Drawing for the job (mm, zero at the part's lowest x, y, z). A direction names the side the tool comes from. Round coordinates to 2 decimals unless told otherwise and drop trailing zeros. Write each loop counter-clockwise with the first axis right and the second up, starting at its lowest first coordinate (ties: lowest second). Pieces come first, ordered by that corner, then holes.
Item 1: Band-saw the part on C-C, the plane z = 1.25. Write the cut outline in (x, y).
Item 2: Drop flat-ended pins along their axis: pin 1 Ø3 at (y, z) = (3.5, 6) entering from +X; pin 2 Ø1.5 at (x, z) = (3.5, 4.5) entering from -Y; pin 3 Ø3 at (y, z) = (3, 9) entering from -X. Give the stop position or say it passes through.
Item 3: 3-axis set-ups, long thin cutter, end or side, ignore diameter. For the marked faces 1 and 2: which of +Z, -Z, +X, -X, +Y, -Y reach the whole face in a straight line?
Item 4: Band-saw the part on D-D, the plane z = 9.5. Write the cut outline in (x, y), then the cut area to 3 significant figures.
Item 5: Wall check: probe 1 along Z at (x, y) = (1, 1.25); probe 2 along Y at (x, z) = (2.5, 7); probe 3 along X at (y, z) = (1.25, 7). Give the ranges that are in metal, low to high.
Item 6: Band-saw the part on A-A, the plane y = 3.25. Write the cut outline in (x, z).
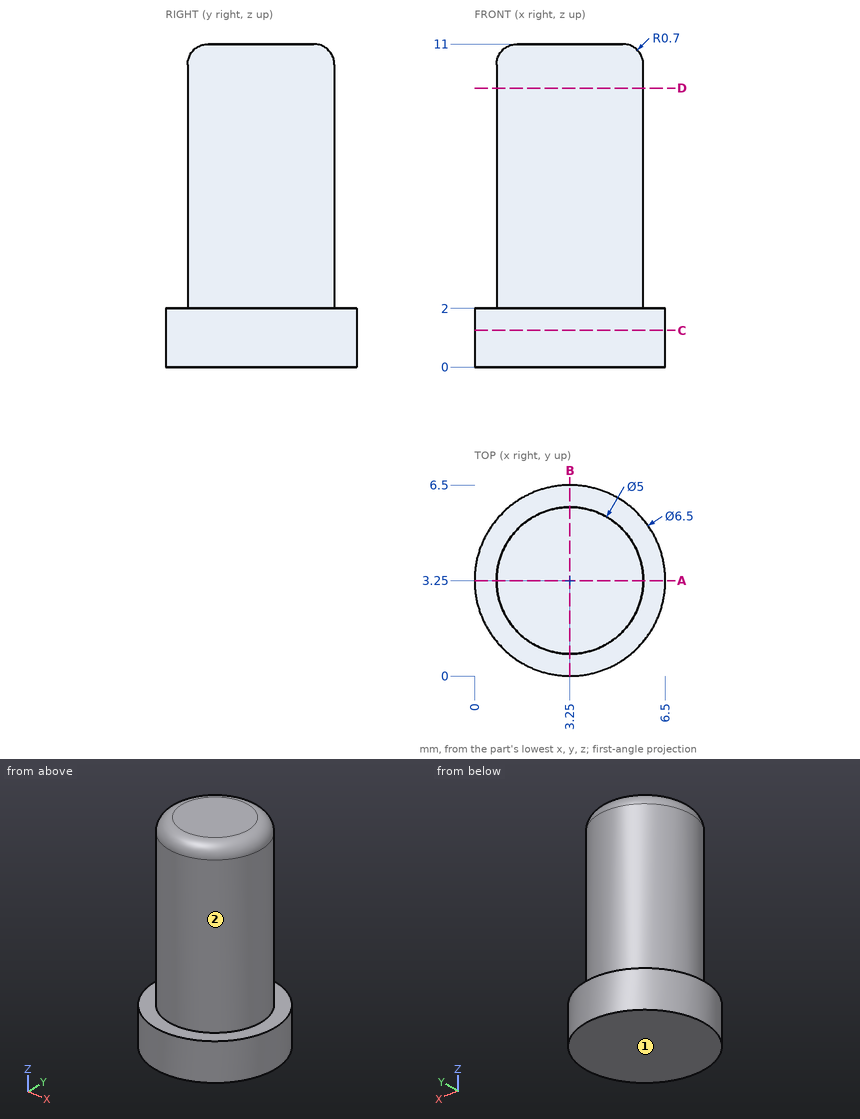
Results:
1. outline: circle Ø6.5 at (3.25, 3.25)
2. pin 1: stops at x = 5.75
2. pin 2: stops at y = 0.75
2. pin 3: stops at x = 0.75
3. face 1: -Z, +X, -X, +Y, -Y
3. face 2: +Z
4. outline: circle Ø5 at (3.25, 3.25)
4. area: 19.6 mm2
5. probe 1: z = 0 to 2
5. probe 2: y = 0.87 to 5.63
5. probe 3: x = 1.75 to 4.75
6. outline: (0, 0) - (6.5, 0) - (6.5, 2) - (5.75, 2) - (5.75, 10.3) arc R0.7 ccw to (5.05, 11) - (1.45, 11) arc R0.7 ccw to (0.75, 10.3) - (0.75, 2) - (0, 2) - close
